Verification items for the finished model (mm, model axes). A direction names the side the tool comes from. Round coordinates to 2 decimals unless told otherwise and drop trailing zeros. Order: outer loops, then holes, each group sorted by start corner. A loop starts at its lowest first (then second) coordinate and runs counter-clockwise, first axis right, second up. Notation, with made-up numbers: (64.5, -24.5) -> (86.5, -24.5) arc R19 cw to (86.5, -10.5) -> close; hole circle Ø10 at (51, 69). An arc over 180 degrees is marked (long way). Return JSON: item names as keys, results as strings. Group by question number.
Item 1: Scan lines: probe 1 along Y at (x, z) = (4.5, 21); probe 2 along X at (y, z) = (-6.5, 10.5); probe 3 along Z at (x, y) = (30, -1.5). Record each from-to range of solid material in increasing order. Write a range as from..to.
Item 2: Sectioned sample at B-B on x = 6.5. Record the cut outline in (y, z), plus the area to 3 significant figures.
Item 3: Sectioned sample at A-A on y = 9.5. Record the cut outline in (x, z), plus the area to 3 significant figures.
Item 4: Sectioned sample at C-C on z = 22. Record the cut outline in (x, y).
Item 5: Access from +Z, -Z, +X, -X, +Y, -Y to the whole of each face (thin tool, end or side, straight path). Record for faces 1 (the flat face through (12, 12.7, 22)), 2 (the flat face through (24, 16, 31.75)).
```python
from build123d import *

# Parameters (mm, degrees)
F0_W     = 38.1
F0_H     = 25.4
F2_DEPTH = 31.75
F4_DEPTH = 12.7
F5_DEPTH = 8.89


with BuildPart() as f2:
    # F0 (on Top) → F2 (new body)
    with BuildSketch(Plane.XY):
        with Locations((19.05, 12.7)):
            Rectangle(F0_W, F0_H)
    extrude(amount=F2_DEPTH)

    # F3 (on face) → F4 (cut)
    with BuildSketch(Plane.XZ):
        Polygon((0, 31.75), (0, 6.521496), (31.439457, 31.75), align=None)
    extrude(amount=-F4_DEPTH, mode=Mode.SUBTRACT)

    # F2_face (on face) → F5 (join)
    with BuildSketch(Plane(origin=(19.05, 0, 15.875), x_dir=(1, 0, 0), z_dir=(0, -1, 0))):
        Polygon((-19.05, -15.875), (19.05, -15.875), (19.05, 15.875), (12.389457, 15.875), (-19.05, -9.353504), align=None)
    extrude(amount=F5_DEPTH)


solid = f2.part
```
Recorded:
{
 "1": {"probe 1": "12.7..25.4", "probe 2": "4.96..38.1", "probe 3": "0..30.59"},
 "2": {"outline": "(-8.89, 0) -> (25.4, 0) -> (25.4, 31.75) -> (12.7, 31.75) -> (12.7, 11.74) -> (-8.89, 11.74) -> close", "area": "657 mm²"},
 "3": {"outline": "(0, 0) -> (38.1, 0) -> (38.1, 31.75) -> (31.44, 31.75) -> (0, 6.52) -> close", "area": "813 mm²"},
 "4": {"outline": "(0, 12.7) -> (19.29, 12.7) -> (19.29, -8.89) -> (38.1, -8.89) -> (38.1, 25.4) -> (0, 25.4) -> close"},
 "5": {"face 1": "+Z, -X, -Y", "face 2": "+Z, +X, -X, +Y, -Y"}
}
